```python
from build123d import *

# Parameters (mm, degrees)
SKETCH1_W           = 38
SKETCH1_H           = 38
BOSS_EXTRUDE1_DEPTH = 33
SKETCH2_R           = 2.2
BOSS_EXTRUDE2_DEPTH = 33
FILLET1_R           = 3
SKETCH3_R           = 1.25
CUT_EXTRUDE1_DEPTH  = 7


with BuildPart() as part:
    # Sketch1 → Boss-Extrude1 (new body)
    with BuildSketch(Plane(origin=(0, 0, 0), x_dir=(1, 0, 0), z_dir=(0, 1, 0))):
        with Locations((19, 19)):
            Rectangle(SKETCH1_W, SKETCH1_H)
    extrude(amount=BOSS_EXTRUDE1_DEPTH)

    # Sketch2 → Boss-Extrude2 (add)
    with BuildSketch(Plane(origin=(0, 33, 0), x_dir=(1, 0, 0), z_dir=(0, 1, 0))):
        with Locations(Location((19, 19.398847775, 0), (0, 0, 270))):
            Circle(SKETCH2_R)
    extrude(amount=BOSS_EXTRUDE2_DEPTH)

    # Fillet1
    fillet1_edges = [part.edges().sort_by_distance(p)[0] for p in [
        (38, 16.5, -38),
        (38, 16.5, 0),
        (0, 16.5, 0),
        (0, 16.5, -38),
    ]]
    fillet(fillet1_edges, radius=FILLET1_R)

    # Sketch3 → Cut-Extrude1 (cut)
    with BuildSketch(Plane(origin=(0, 33, 0), x_dir=(1, 0, 0), z_dir=(0, 1, 0))):
        with Locations(Location((3.5, 34.5, 0), (0, 0, 270))):
            Circle(SKETCH3_R)
        with Locations(Location((3.5, 3.5, 0), (0, 0, 270))):
            Circle(SKETCH3_R)
        with Locations(Location((34.5, 3.5, 0), (0, 0, 270))):
            Circle(SKETCH3_R)
        with Locations(Location((34.5, 34.5, 0), (0, 0, 270))):
            Circle(SKETCH3_R)
    extrude(amount=-CUT_EXTRUDE1_DEPTH, mode=Mode.SUBTRACT)


solid = part.part
```
Verification items for the finished model (mm, model axes). A direction names the side the tool comes from. Coordinates: 2 decimals unless noted, no trailing zeros. Loops run counter-clockwise (first coordinate to the right, second up) from the corner with the lowest first, then second, coordinate; pieces in that order, holes last. Notation, with made-up numbers: (21, 26) - (74, 26) arc R8 cw to (74, 31) - close; hole circle Ø3 at (4.25, 80). An arc over 180 degrees is marked (long way). Return JSON: item names as keys, results as strings.
1. Section check A-A, the plane x = 19. Record the boundary of the cut face in (y, z).
Established:
{"outline": "(0, -38) - (33, -38) - (33, -21.6) - (66, -21.6) - (66, -17.2) - (33, -17.2) - (33, 0) - (0, 0) - close"}
2. Tool access check on faces 4 (the flat face through (19, 16, -38)), 5 (the cylindrical face through (17.661, 49.269, -21.145)). Record the directions out of +Z, -Z, +X, -X, +Y, -Y that give a thin tool (end or side, any length) a straight path to the whole face; none if there is none.
Established:
{"face 4": "-Z, +X, -X, +Y, -Y", "face 5": "+Y"}
3. Section check B-B, the plane y = 28. Record the boundary of the cut face in (x, z), then the cut area to 3 significant figures.
Established:
{"outline": "(0, -35) arc R3 ccw to (3, -38) - (35, -38) arc R3 ccw to (38, -35) - (38, -3) arc R3 ccw to (35, 0) - (3, 0) arc R3 ccw to (0, -3) - close; hole circle Ø2.5 at (3.5, -34.5); hole circle Ø2.5 at (3.5, -3.5); hole circle Ø2.5 at (34.5, -34.5); hole circle Ø2.5 at (34.5, -3.5)", "area": "1,420 mm2"}
4. Section check D-D, the plane z = -32.5. Record the boundary of the cut face in (x, y).
Established:
{"outline": "(0, 0) - (38, 0) - (38, 33) - (0, 33) - close"}
5. Section check C-C, the plane y = 61.5. Record the boundary of the cut face in (x, z), then the cut area to 3 significant figures.
Established:
{"outline": "circle Ø4.4 at (19, -19.4)", "area": "15.2 mm2"}
6. Mould release check, pull along Z, two halves, no side actions. Record for faces 1 (the flat face through (38, 16, -19)), 2 (the cylindrical face through (37.1, 16.73, -0.86)), 3 (the flat face through (4, 26, -35)): +Z half, -Z half, draft (parallel to the pull), parting line (faces both ways), or undercut.
Established:
{"face 1": "draft", "face 2": "+Z half", "face 3": "undercut"}
7. Go/stop test with flat-tipped pins: pin 1 (0.8 mm diameter, centred on x = 4, z = -35, fed in from +Y); pin 2 (3 mm diameter, centred on y = 47.5, z = -22, fed in from -X); pin 3 (2 mm diameter, centred on x = 3, z = -3, fed in from +Y). Record where each tip stops, or that it passes through.
Established:
{"pin 1": "stops at y = 26", "pin 2": "stops at x = 17.1", "pin 3": "stops at y = 33"}
8. Thickness scan on L1, parallel to X at y = 29.25, z = -34.5; L2, parallel to Y at x = 5, z = -26; L3, parallel to Z at x = 20, y = 62. Record the ranges inside material, lowest first.
Established:
{"L1": "x = 0 to 2.25, 4.75 to 33.25, 35.75 to 38", "L2": "y = 0 to 33", "L3": "z = -21.36 to -17.44"}
